Here's the drawing with two shaded views (mm, measured from the low corner). I have some questions. Coordinates: 2 decimals unless noted, no trailing zeros. Loops run counter-clockwise (first coordinate to the right, second up) from the corner with the lowest first, then second, coordinate; pieces in that order, holes last. Notation, with made-up numbers: (53, 48.25) -> (62, 48.25) arc R27 cw to (62, 70.25) -> close; hole circle Ø2 at (18, 51). An arc over 180 degrees is marked (long way). Answer as a JSON object with one key per item and string values. Group by question number.
Q1. I need wall thicknesses on line 1 (Y direction, x = 30, z = 16); line 2 (Z direction, x = 29, y = 56); line 3 (Y direction, x = 11.5, z = 595). Which ranges of each line are inside material? Lowest first, please.
Q2. I want a section at B-B on y = 160. Write out the boundary of the cut face in (x, z).
Q3. I want a section at A-A on z = 690. Write out the boundary of the cut face in (x, y), then the cut area to 3 significant figures.
Q4. Thinking about a two-plate mould opening in Z: for the marked faces 1 and 2, which applies, released by +Z, released by -Z, zero draft, split by the parting line, or undercut?
Q5. I want a section at D-D on y = 50. Write out the boundary of the cut face in (x, z).
Q6. I want a section at C-C on x = 30. Write out the boundary of the cut face in (y, z), then the cut area to 3 significant figures.
Q7. I'm going to push flat-ended pins straight in: pin 1 (16.5 mm diameter, centred on x = 30, z = 688, fed in from -Y); pin 2 (6 mm diameter, centred on x = 39, y = 200.5, fed in from +Z); pin 3 (2 mm diameter, centred on x = 19, y = 37.5, fed in from +Z). Where does each tip first touch, or does it pass through?
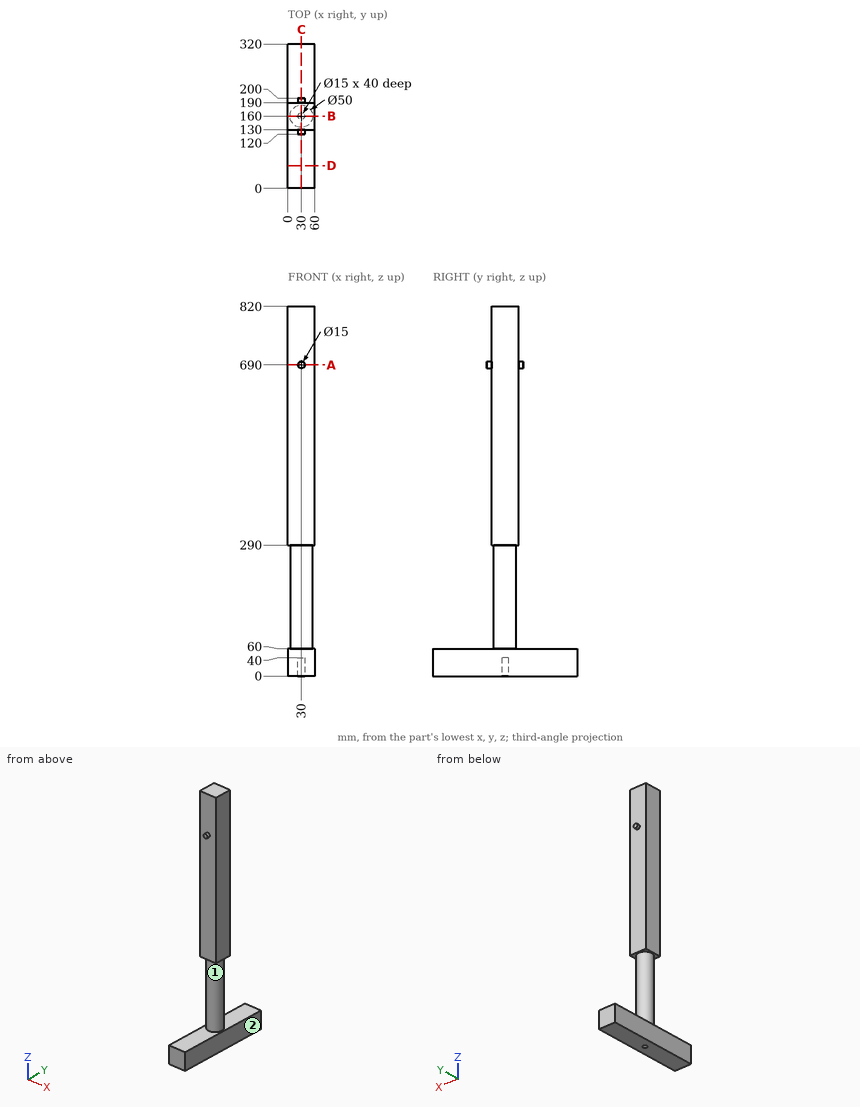
Result set:
{
 "1": {"line 1": "y = 0 to 152.5, 167.5 to 320", "line 2": "z = 0 to 60", "line 3": "y = 130 to 190"},
 "2": {"outline": "(0, 0) -> (22.5, 0) -> (22.5, 40) -> (37.5, 40) -> (37.5, 0) -> (60, 0) -> (60, 60) -> (55, 60) -> (55, 290) -> (60, 290) -> (60, 820) -> (0, 820) -> (0, 290) -> (5, 290) -> (5, 60) -> (0, 60) -> close"},
 "3": {"outline": "(0, 130) -> (22.5, 130) -> (22.5, 120) -> (37.5, 120) -> (37.5, 130) -> (60, 130) -> (60, 190) -> (37.5, 190) -> (37.5, 200) -> (22.5, 200) -> (22.5, 190) -> (0, 190) -> close", "area": "3,900 mm²"},
 "4": {"face 1": "undercut", "face 2": "zero draft"},
 "5": {"outline": "(0, 0) -> (60, 0) -> (60, 60) -> (0, 60) -> close"},
 "6": {"outline": "(0, 0) -> (152.5, 0) -> (152.5, 40) -> (167.5, 40) -> (167.5, 0) -> (320, 0) -> (320, 60) -> (185, 60) -> (185, 290) -> (190, 290) -> (190, 682.5) -> (200, 682.5) -> (200, 697.5) -> (190, 697.5) -> (190, 820) -> (130, 820) -> (130, 697.5) -> (120, 697.5) -> (120, 682.5) -> (130, 682.5) -> (130, 290) -> (135, 290) -> (135, 60) -> (0, 60) -> close", "area": "62,200 mm²"},
 "7": {"pin 1": "stops at y = 120", "pin 2": "stops at z = 694.44", "pin 3": "stops at z = 60"}
}
